```python
from build123d import *

# Parameters (mm, degrees)
SKETCH1_R               = 92.075
BOSS_EXTRUDE1_DEPTH     = 6.35
BOSS_EXTRUDE4_START     = 94.615
SKETCH2_W               = 25.4
SKETCH2_H               = 44.45
BOSS_EXTRUDE4_DEPTH     = 6.35
SKETCH4_R               = 2.1463
CUT_EXTRUDE2_DEPTH      = 6.35
CIRPATTERN1_COUNT       = 3
SKETCH3_R               = 89.8525
CUT_EXTRUDE1_DEPTH      = 50.8
CUT_EXTRUDE1_DEPTH_BACK = 6.35


with BuildPart() as part:
    # Sketch1 → Boss-Extrude1 (new body)
    with BuildSketch(Plane(origin=(0, 0, 0), x_dir=(1, 0, 0), z_dir=(0, 1, 0))):
        Circle(SKETCH1_R)
    extrude(amount=BOSS_EXTRUDE1_DEPTH)

    # Sketch2 → Boss-Extrude4 (add)
    with BuildSketch(Plane.XY.offset(BOSS_EXTRUDE4_START)):
        with Locations((0, 22.225)):
            Rectangle(SKETCH2_W, SKETCH2_H)
    boss_extrude4 = extrude(amount=-BOSS_EXTRUDE4_DEPTH)

    # Sketch4 → Cut-Extrude2 (cut)
    with BuildSketch(Plane.XY.offset(94.615)):
        with Locations((0, 38.1)):
            Circle(SKETCH4_R)
        with Locations((0, 22.225)):
            Circle(SKETCH4_R)
        with Locations((0, 6.35)):
            Circle(SKETCH4_R)
    cut_extrude2 = extrude(amount=-CUT_EXTRUDE2_DEPTH, mode=Mode.SUBTRACT)

    # CirPattern1: Boss-Extrude4, Cut-Extrude2 ×3 about axis
    cirpattern1_axis = Axis((0, 0, 0), (0, 1, 0))
    for i in range(1, CIRPATTERN1_COUNT):
        add(boss_extrude4.rotate(cirpattern1_axis, i * 360 / CIRPATTERN1_COUNT))
        add(cut_extrude2.rotate(cirpattern1_axis, i * 360 / CIRPATTERN1_COUNT), mode=Mode.SUBTRACT)

    # Sketch3 → Cut-Extrude1 (cut, two sides)
    with BuildSketch(Plane(origin=(0, 6.35, 0), x_dir=(1, 0, 0), z_dir=(0, 1, 0))) as cut_extrude1_sk:
        Circle(SKETCH3_R)
    extrude(amount=CUT_EXTRUDE1_DEPTH, mode=Mode.SUBTRACT)
    extrude(cut_extrude1_sk.sketch, amount=-CUT_EXTRUDE1_DEPTH_BACK, mode=Mode.SUBTRACT)


solid = part.part
```
Here's how the part is built. I have some questions about the finished solid (model axes, mm). A direction names the side the tool comes from. Round coordinates to 2 decimals unless told otherwise and drop trailing zeros. Write each loop counter-clockwise with the first axis right and the second up, starting at its lowest first coordinate (ties: lowest second). Pieces come first, ordered by that corner, then holes.
Q1. If we section it at D-D on x = -68.5: Write out the boundary of the cut face in (y, z).
Q2. If we section it at A-A on y = 28: Write out the boundary of the cut face in (x, z) (1 decimal), plus the area to 3 significant figures.
Q3. Please list where these lines run through material, in increasing order: probe 1 along Y at (x, z) = (0, 91); probe 2 along X at (y, z) = (38, 91); probe 3 along Z at (x, y) = (0, 1.5) (1 decimal).
Q4. Which directions (+Z, -Z, +X, -X, +Y, -Y) give clear straight access to the entire face, cutting with the end or side of a thin tool? Please do faces 5 (the cylindrical face through (-0.465, 4.255, 92.254)), 6 (the cylindrical face through (1.171, 3.131, -92.068)), 7 (the flat face through (73.17, 21.91, -56.91)).
Q5. If we section it at B-B on x = 0: Give the number of separate pieces and of enclosed holes in the cut face, plus the area to 3 significant figures.
Q6. Will these pins go through, and if not, where does the flat tip stop? P1, Ø8, axis at y = 22.5, z = -42.5, coming from the -X side; P2, Ø6, axis at y = 32, z = 91.5, coming from the +X side; P3, Ø6, axis at x = 47, y = 12, coming from the -Z side; P4, Ø1.5, axis at x = 46, y = 6.5, coming from the +Z side.
Q7. If we mould it in two halves opening along Z, with no side actions, what happens to faces 1 (the cylindrical face through (-80.47, 39.91, -45.13)), 2 (the flat face through (12.7, 22, 92)), 3 (the flat face through (3, 23, 94.615)), 4 (the flat face through (-73.17, 21.91, -56.91))? For each: +Z half, -Z half, draft (parallel to the pull), parting line (faces both ways), or undercut.
Answer below:
1. outline: (0, -61.53) - (6.35, -61.53) - (6.35, -58.15) - (0, -58.15) - close; (0, 58.15) - (6.35, 58.15) - (6.35, 61.53) - (0, 61.53) - close
2. outline: (-88.3, -36.3) - (-75.6, -58.3) - (-70.7, -55.5) arc R89.9 cw to (-83.4, -33.5) - close; (-12.7, 89) arc R89.9 cw to (12.7, 89) - (12.7, 94.6) - (-12.7, 94.6) - close; (70.7, -55.5) - (75.6, -58.3) - (88.3, -36.3) - (83.4, -33.5) arc R89.9 cw to start
2. area: 386 mm2
3. probe 1: y = 0 to 4.2, 8.5 to 20.08, 24.37 to 35.95, 40.25 to 44.45
3. probe 2: x = -12.7 to -2.14, 2.14 to 12.7
3. probe 3: z = -92.1 to -89.9, 89.9 to 94.6
4. face 5: +Z
4. face 6: -Z, +Y, -Y
4. face 7: -Z, +Y
5. separate pieces: 5
5. enclosed holes: 0
5. area: 164 mm2
6. P1: stops at x = -87.02
6. P2: stops at x = 12.7
6. P3: passes through
6. P4: stops at z = 80.18
7. face 1: undercut
7. face 2: draft
7. face 3: +Z half
7. face 4: -Z half
